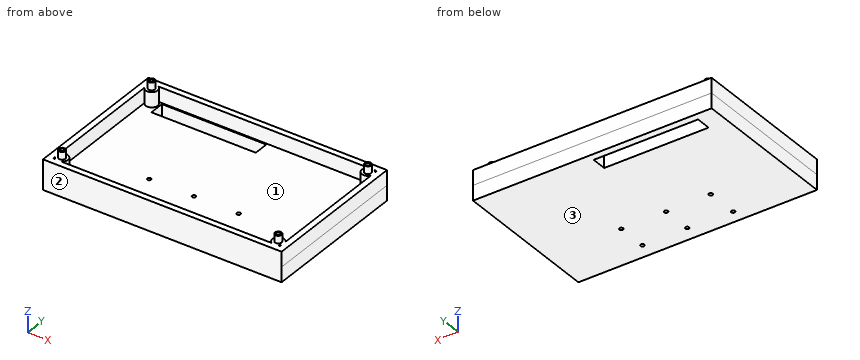
from build123d import *

# Parameters (mm, degrees)
SKETCH2_W                 = 101.6
SKETCH2_H                 = 63.5
BOSS_EXTRUDE1_DEPTH       = 6.35
SKETCH3_R                 = 2.54
BOSS_EXTRUDE2_DEPTH       = 6.35
SKETCH4_R                 = 1.397
BOSS_EXTRUDE3_DEPTH       = 3.175
M2X0_4_TAPPED_HOLE1_D     = 1.6
M2X0_4_TAPPED_HOLE1_DEPTH = 5.2639976
M2X0_4_TAPPED_HOLE1_TIP   = 0.480688495
SKETCH8_W                 = 44.45
SKETCH8_H                 = 6.35
CUT_EXTRUDE1_DEPTH        = 8.255
BOSS_EXTRUDE5_DEPTH       = 6.35
M2X0_4_TAPPED_HOLE2_D     = 1.6


with BuildPart() as part:
    # Sketch2 → Boss-Extrude1 (new body)
    with BuildSketch(Plane.XY):
        with Locations((50.8, 31.75)):
            Rectangle(SKETCH2_W, SKETCH2_H)
    extrude(amount=BOSS_EXTRUDE1_DEPTH)

    # Sketch3 → Boss-Extrude2 (add)
    with BuildSketch(Plane.XY.offset(6.35)):
        with Locations(Location((4.7625, 4.7625, 0), (0, 0, 180))):
            Circle(SKETCH3_R)
        with Locations(Location((96.8375, 4.7625, 0), (0, 0, 180))):
            Circle(SKETCH3_R)
        with Locations(Location((96.8375, 58.7375, 0), (0, 0, 180))):
            Circle(SKETCH3_R)
        with Locations(Location((4.7625, 58.7375, 0), (0, 0, 180))):
            Circle(SKETCH3_R)
    extrude(amount=BOSS_EXTRUDE2_DEPTH)

    # Sketch4 → Boss-Extrude3 (add)
    with BuildSketch(Plane.XY.offset(12.7)):
        with Locations((4.7625, 58.7375)):
            Circle(SKETCH4_R)
        with Locations((4.7625, 4.7625)):
            Circle(SKETCH4_R)
        with Locations((96.8375, 58.7375)):
            Circle(SKETCH4_R)
        with Locations((96.8375, 4.7625)):
            Circle(SKETCH4_R)
    extrude(amount=BOSS_EXTRUDE3_DEPTH)

    # M2x0.4 Tapped Hole1
    with Locations(Plane.XY.offset(15.875)):
        with Locations((4.7625, 58.7375), (4.7625, 4.7625), (96.8375, 58.7375), (96.8375, 4.7625)):
            Hole(M2X0_4_TAPPED_HOLE1_D / 2, depth=M2X0_4_TAPPED_HOLE1_DEPTH)
            with Locations((0, 0, -(M2X0_4_TAPPED_HOLE1_DEPTH + M2X0_4_TAPPED_HOLE1_TIP / 2))):  # 118° drill point
                Cone(0, M2X0_4_TAPPED_HOLE1_D / 2, M2X0_4_TAPPED_HOLE1_TIP, mode=Mode.SUBTRACT)

    # Sketch8 → Cut-Extrude1 (cut)
    with BuildSketch(Plane.XY.offset(6.35)):
        with Locations((30.1625, 57.253105079)):
            Rectangle(SKETCH8_W, SKETCH8_H)
    extrude(amount=-CUT_EXTRUDE1_DEPTH, mode=Mode.SUBTRACT)

    # 3DSketch1 → Boss-Extrude5 (add)
    with BuildSketch(Plane(origin=(2.54, 2.54, 6.35), x_dir=(0.851658316704544, 0.5240974256643347, 0), z_dir=(0, 0, -1))):
        Polygon((83.034065392, 54.080303111), (116.314251921, 0), (29.785766944, -53.248298447), (-3.494419586, 0.832004663), align=None)
        Polygon((0, 0), (82.202060728, 50.585883525), (112.819832336, 0.832004663), (30.617771607, -49.753878862), align=None, mode=Mode.SUBTRACT)
    extrude(amount=-BOSS_EXTRUDE5_DEPTH)

    # M2x0.4 Tapped Hole2 (through all)
    with Locations(Plane(origin=(0, 0, 0), x_dir=(-1, 0, 0), z_dir=(0, 0, -1))):
        with Locations((-69.85, 19.05), (-50.8, 19.05), (-31.75, 19.05), (-69.85, 6.35), (-50.8, 6.35), (-31.75, 5.62052836)):
            Hole(M2X0_4_TAPPED_HOLE2_D / 2)


solid = part.part
The listing builds one solid part. Answer for the finished solid, in the listing's coordinates (mm). Face numbers are marked on the shaded views. Round coordinates to 2 decimals unless told otherwise and drop trailing zeros. Loops run counter-clockwise (first coordinate to the right, second up) from the corner with the lowest first, then second, coordinate; pieces in that order, holes last. Notation, with made-up numbers: M 63.5,77.25 L 68.5,77.25 A14 ccw 68.5,89.25 Z; hole C 76.5,45.5 d11. An arc over 180 degrees is marked long. Return JSON: item names as keys, results as strings.
Q1. Find section A-A, the plane x = 23.5. Determine the outline of the cut face in (y, z), plus the area to 3 significant figures.
Results list:
{"outline": "M 0,0 L 54.08,0 L 54.08,6.35 L 2.54,6.35 L 2.54,12.7 L 0,12.7 Z; M 60.43,0 L 63.5,0 L 63.5,12.7 L 60.96,12.7 L 60.96,6.35 L 60.43,6.35 Z", "area": "395 mm2"}
Q2. Find the intervals of material crossed by line 1 along Y through (x, z) = (50.8, 4); line 2 along Y through (x, z) = (31.75, 2.5); line 3 along X through (y, z) = (13.5, 12), in increasing order. Write a range as from..to.
Results list:
{"line 1": "y = 0..5.55, 7.15..18.25, 19.85..54.08, 60.43..63.5", "line 2": "y = 0..4.82, 6.42..18.25, 19.85..54.08, 60.43..63.5", "line 3": "x = 0..2.54, 99.06..101.6"}
Q3. Find section C-C, the plane z = 3.5. Determine the outline of the cut face in (x, y), plus the area to 3 significant figures.
Results list:
{"outline": "M 0,0 L 101.6,0 L 101.6,63.5 L 0,63.5 Z; hole M 7.94,54.08 L 52.39,54.08 L 52.39,60.43 L 7.94,60.43 Z; hole C 31.75,5.62 d1.6; hole C 31.75,19.05 d1.6; hole C 50.8,6.35 d1.6; hole C 50.8,19.05 d1.6; hole C 69.85,6.35 d1.6; hole C 69.85,19.05 d1.6", "area": "6,160 mm2"}
Q4. Find section D-D, the plane y = 26.5. Determine the outline of the cut face in (x, z).
Results list:
{"outline": "M 0,0 L 101.6,0 L 101.6,12.7 L 99.06,12.7 L 99.06,6.35 L 2.54,6.35 L 2.54,12.7 L 0,12.7 Z"}
Q5. Find section B-B, the plane x = 92.5. Determine the outline of the cut face in (y, z), plus the area to 3 significant figures.
Results list:
{"outline": "M 0,0 L 63.5,0 L 63.5,12.7 L 60.96,12.7 L 60.96,6.35 L 2.54,6.35 L 2.54,12.7 L 0,12.7 Z", "area": "435 mm2"}
Q6. The mould has two halves that part along Y. Classify the marked faces 1, 2 and 3: released by +Y, released by -Y, zero draft, split by the parting line, or undercut.
Results list:
{"face 1": "undercut", "face 2": "released by -Y", "face 3": "zero draft"}
Q7. Each of these flat-tipped pins is pushed along its axis until it touches: pin 1 Ø8 at (x, y) = (86.5, 37) entering from -Z; pin 2 Ø1.1 at (x, y) = (3, 60.5) entering from +Z; pin 3 Ø1.3 at (x, y) = (4.76, 4.76) entering from +Z; pin 4 Ø1 at (x, y) = (4.76, 58.74) entering from +Z. Where does it stop, or does it pass through?
Results list:
{"pin 1": "stops at z = 0", "pin 2": "stops at z = 12.7", "pin 3": "stops at z = 10.52", "pin 4": "stops at z = 10.43"}
